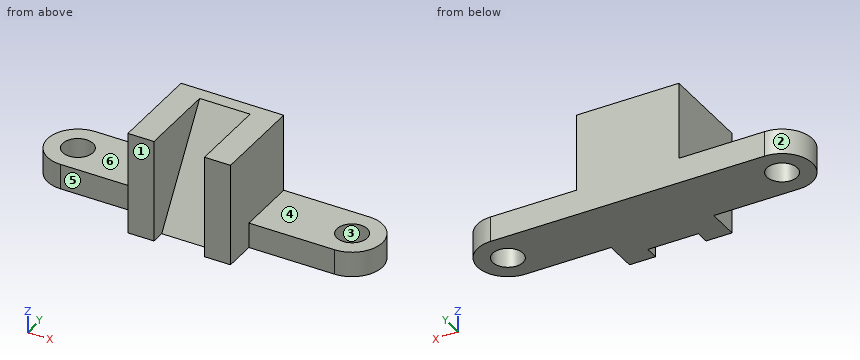
```python
from build123d import *

# Parameters (mm, degrees)
F0_W     = 61
F0_H     = 55
F1_DEPTH = 61
F2_W     = 30
F2_H     = 47.25
F3_DEPTH = 61
F4_R     = 9
F5_DEPTH = 15
F7_DEPTH = 30


with BuildPart() as f1:
    # F0 (on Top) → F1 (new body)
    with BuildSketch(Plane.XY):
        Rectangle(F0_W, F0_H)
    extrude(amount=F1_DEPTH)

    # F2 (on face) → F3 (cut)
    with BuildSketch(Plane.XY.offset(61)):
        with Locations((0, -3.875)):
            Rectangle(F2_W, F2_H)
    extrude(amount=-F3_DEPTH, mode=Mode.SUBTRACT)

    # F4 (on face) → F5 (join)
    with BuildSketch(Plane(origin=(0, 0, 0), x_dir=(1, 0, 0), z_dir=(0, 0, -1))):
        with BuildLine():
            Line((-81.5, -27.5), (-30.5, -27.5))
            Line((-30.5, -27.5), (-30.5, 8.5))
            Line((-30.5, 8.5), (-81.5, 8.5))
            ThreePointArc((-81.5, 8.5), (-99.5, -9.5), (-81.5, -27.5))
        make_face()
        with Locations((-81.5, -9.5)):
            Circle(F4_R, mode=Mode.SUBTRACT)
        with BuildLine():
            Line((30.5, 8.5), (30.5, -27.5))
            Line((30.5, -27.5), (81.5, -27.5))
            ThreePointArc((81.5, -27.5), (99.5, -9.5), (81.5, 8.5))
            Line((81.5, 8.5), (30.5, 8.5))
        make_face()
        with Locations((81.5, -9.5)):
            Circle(F4_R, mode=Mode.SUBTRACT)
    extrude(amount=-F5_DEPTH)

    # F6 (on face) → F7 (join)
    with BuildSketch(Plane.YZ.offset(-15)):
        Polygon((19.75, 0), (19.75, 61), (-19.5, 0), align=None)
    extrude(amount=F7_DEPTH)


solid = f1.part
```
Can you work these out from the model? Positions are in its coordinate system, mm. Face numbers are marked on the shaded views. A direction names the side the tool comes from. Give positions to 0.01 mm unless a question says otherwise; leave off trailing zeros. Loops run counter-clockwise (first coordinate to the right, second up) from the corner with the lowest first, then second, coordinate; pieces in that order, holes last. Notation, with made-up numbers: M 40.5,41.5 L 59.5,41.5 A21 ccw 59.5,48.5 Z; hole C -34.5,-39 d1. An arc over 180 degrees is marked long. Use CSV: the item, a comma, the result in double quotes. Start each with the question number.
1. Imagine slicing it at A-A, the plane y = -23. Write out the boundary of the cut face in (x, z), plus the area to 3 significant figures.
2. If I drill on L1, parallel to X at y = 9.5, z = 11.25; L2, parallel to Y at x = 81.5, z = 7; L3, parallel to X at y = -10, z = 46, over which ranges is the centre line in solid material (lowest first)?
3. Imagine slicing it at B-B, the plane y = 9.5. Write out the boundary of the cut face in (x, z).
4. On a 3-axis mill with a long thin cutter (end or side, diameter ignored), from which of +Z, -Z, +X, -X, +Y, -Y can I reach the whole of each face in a straight line? I mean the marked faces 4, 5 and 6. Say none if no direction works.
5. Imagine slicing it at D-D, the plane x = 8. Write out the boundary of the cut face in (y, z).
6. Imagine slicing it at C-C, the plane z = 10. Write out the boundary of the cut face in (x, y), plus the area to 3 significant figures.
7. If we mould it in two halves opening along X, with no side actions, what happens to the marked faces 1, 2 and 3? For each: released by +X, released by -X, zero draft, split by the parting line, or undercut.
8. For P1, Ø16.5, axis at y = -8, z = 21.5, coming from the -X side; P2, Ø4.5, axis at x = -57.5, z = 9, coming from the -Y side; P3, Ø8, axis at y = -0.5, z = 52.5, coming from the -X side; P4, Ø14.5, axis at x = 81.5, y = 9.5, coming from the +Z side, each with a flat end and sliding along its axis, tell me the tip position at first contact or that it passes through.
Response values:
1,outline,"M -30.5,0 L -15,0 L -15,61 L -30.5,61 Z; M 15,0 L 30.5,0 L 30.5,61 L 15,61 Z"
1,area,"1,890 mm^2"
2,L1,"-99.5 to -90.5, -72.5 to 72.5, 90.5 to 99.5"
2,L2,"-8.5 to 0.5, 18.5 to 27.5"
2,L3,"-30.5 to -15, 15 to 30.5"
3,outline,"M -99.5,0 L -90.5,0 L -90.5,15 L -99.5,15 Z; M -72.5,0 L 72.5,0 L 72.5,15 L 30.5,15 L 30.5,61 L 15,61 L 15,45.07 L -15,45.07 L -15,61 L -30.5,61 L -30.5,15 L -72.5,15 Z; M 90.5,0 L 99.5,0 L 99.5,15 L 90.5,15 Z"
4,face 4,"+Z, +X, +Y, -Y"
4,face 5,"+Z, -Z, -X, -Y"
4,face 6,"+Z, -X, +Y, -Y"
5,outline,"M -19.5,0 L 27.5,0 L 27.5,61 L 19.75,61 Z"
6,outline,"M -81.5,-8.5 L -30.5,-8.5 L -30.5,-27.5 L -15,-27.5 L -15,-13.07 L 15,-13.07 L 15,-27.5 L 30.5,-27.5 L 30.5,-8.5 L 81.5,-8.5 A18 ccw 81.5,27.5 L -81.5,27.5 A18 ccw Z; hole C -81.5,9.5 d18; hole C 81.5,9.5 d18"
6,area,"7,100 mm^2"
7,face 1,"zero draft"
7,face 2,"released by -X"
7,face 3,"undercut"
8,P1,"x = -94.53"
8,P2,"y = -8.5"
8,P3,"x = -30.5"
8,P4,"through"
